Here's how the part is built. I have some questions about the finished solid (model axes, mm). Give positions to 0.01 mm unless a question says otherwise; leave off trailing zeros. Write each loop counter-clockwise with the first axis right and the second up, starting at its lowest first coordinate (ties: lowest second). Pieces come first, ordered by that corner, then holes. Notation, with made-up numbers: (56, -34) -> (110, -34) arc R22 cw to (110, -12) -> close; hole circle Ø5 at (-6.5, 80.25). An arc over 180 degrees is marked (long way). Return JSON: item names as keys, results as strings.
from build123d import *

# Parameters (mm, degrees)
BOSS_EXTRUDE1_DEPTH      = 98.610323
BOSS_EXTRUDE1_DEPTH_BACK = 87.674643
SKETCH1_R                = 7.9375
SKETCH1_R_2              = 6.4643
CUT_EXTRUDE1_DEPTH       = 101.194886763
FILLET1_R                = 1.5875


with BuildPart() as part:
    # Sketch1 → Boss-Extrude1 (new, two sides: drawn at the far end of the back side and taken through both)
    with BuildSketch(Plane(origin=(0, 0, 0), x_dir=(0, 0, -1), z_dir=(1, 0, 0)).offset(-BOSS_EXTRUDE1_DEPTH_BACK)):
        with Locations(Location((0, 0, 0), (0, 0, 180))):
            Circle(SKETCH1_R)
        with Locations(Location((0, 0, 0), (0, 0, 180))):
            Circle(SKETCH1_R_2, mode=Mode.SUBTRACT)
    extrude(amount=BOSS_EXTRUDE1_DEPTH + BOSS_EXTRUDE1_DEPTH_BACK)

    # Sketch2 → Cut-Extrude1 (cut, through all)
    with BuildSketch(Plane(origin=(0, 0, -7.9375), x_dir=(-1, 0, 0), z_dir=(0, 0, -1))):
        Polygon((-55.74782316, -3.175), (-54.16032316, -3.175), (-52.57282316, -3.175), (-52.57282316, 3.175), (-54.16032316, 3.175), (-55.74782316, 3.175), (-106.86532316, 3.175), (-106.86532316, -3.175), align=None)
    extrude(amount=-CUT_EXTRUDE1_DEPTH, mode=Mode.SUBTRACT)

    # Fillet1
    fillet1_edges = [part.edges().sort_by_distance(p)[0] for p in [
        (52.57282316, 3.175, -6.452847911),
        (52.57282316, 3.175, 6.452847911),
        (52.57282316, -3.175, -6.452847911),
        (52.57282316, -3.175, 6.452847911),
    ]]
    fillet(fillet1_edges, radius=FILLET1_R)


solid = part.part
1. Suppose I cut it at C-C, the plane x = 48.5. List the corners of the cut face in (y, z) for me (1 decimal), and give its area (3 significant figures).
Taken from the geometry:
{"outline": "circle Ø15.9 at (0, 0); hole circle Ø12.9 at (0, 0)", "area": "66.7 mm²"}
2. If I drill on line 1 (Y direction, x = -29.5, z = -0.5); line 2 (Y direction, x = 37.5, z = 0); line 3 (Z direction, x = -64, y = -2), over which ranges is the centre line in solid material (lowest first)? Write a range as [from, to].
Taken from the geometry:
{"line 1": "y = [-7.92, -6.44], [6.44, 7.92]", "line 2": "y = [-7.94, -6.46], [6.46, 7.94]", "line 3": "z = [-7.68, -6.15], [6.15, 7.68]"}
3. For pin 1 Ø0.8 at (y, z) = (0, -7) entering from +X; pin 2 Ø0.8 at (x, z) = (68.5, -6.5) entering from -Y; pin 3 Ø5 at (x, z) = (75, 6) entering from +Y, each with a flat end and sliding along its axis, tell me the tip position at first contact or that it passes through.
Taken from the geometry:
{"pin 1": "stops at x = 52.57", "pin 2": "stops at y = -5.08", "pin 3": "stops at y = 7.12"}
4. Suppose I cut it at B-B, the plane z = 0. List the corners of the cut face in (x, y) for me, and give its area (3 significant figures).
Taken from the geometry:
{"outline": "(-87.67, -7.94) -> (98.61, -7.94) -> (98.61, -6.46) -> (-87.67, -6.46) -> close; (-87.67, 6.46) -> (98.61, 6.46) -> (98.61, 7.94) -> (-87.67, 7.94) -> close", "area": "549 mm²"}
5. Suppose I cut it at A-A, the plane y = 0. List the corners of the cut face in (x, z) for me, and give its area (3 significant figures).
Taken from the geometry:
{"outline": "(-87.67, -7.94) -> (52.57, -7.94) -> (52.57, -6.46) -> (-87.67, -6.46) -> close; (-87.67, 6.46) -> (52.57, 6.46) -> (52.57, 7.94) -> (-87.67, 7.94) -> close", "area": "413 mm²"}
6. If we mould it in two halves opening along Z, with no side actions, what happens to faces 1 (the face through (4.16, -0.28, -6.46)), 2 (the face through (98.61, -7, 0)), 3 (the face through (4.16, -0.35, -7.93))? For each: released by +Z, released by -Z, zero draft, split by the parting line, or undercut.
Taken from the geometry:
{"face 1": "undercut", "face 2": "zero draft", "face 3": "split by the parting line"}
